The listing builds one solid part. Answer for the finished solid, in the listing's coordinates (mm). A direction names the side the tool comes from. Give positions to 0.01 mm unless a question says otherwise; leave off trailing zeros. Order: outer loops, then holes, each group sorted by start corner. A loop starts at its lowest first (then second) coordinate and runs counter-clockwise, first axis right, second up. Notation, with made-up numbers: (25, 39) -> (38, 39) arc R18 cw to (38, 57) -> close; hole circle Ø5 at (71.5, -17.75). An arc over 180 degrees is marked (long way). Write item = value, one per line. Start each with the question number.
```python
from build123d import *

# Parameters (mm, degrees)
SKETCH1_W                            = 50.8
SKETCH1_H                            = 50.8
BOSS_EXTRUDE1_DEPTH                  = 73.025
CUT_EXTRUDE1_DEPTH                   = 3.175
SKETCH3_R                            = 55.5625
CUT_EXTRUDE2_DEPTH                   = 103.439887861
F_8_32_TAPPED_HOLE1_D                = 3.4544
F_8_32_TAPPED_HOLE1_DEPTH            = 10.70864
F_8_32_TAPPED_HOLE1_TIP              = 1.037806461
F_8_32_TAPPED_HOLE2_D                = 3.4544
F_8_32_TAPPED_HOLE2_DEPTH            = 10.70864
F_8_32_TAPPED_HOLE2_TIP              = 1.037806461
F_10_0_1935_DIAMETER_HOLE1_OUTLINE_R = 2.45745
F_10_0_1935_DIAMETER_HOLE1_DEPTH     = 69.85


# Read off the part's stored shape, not the designer's step: #10 (0.1935) Diameter Hole1
with BuildPart() as part:
    # Sketch1 → Boss-Extrude1 (new body)
    with BuildSketch(Plane(origin=(0, 0, 0), x_dir=(1, 0, 0), z_dir=(0, 1, 0))):
        with Locations((25.4, 25.4)):
            Rectangle(SKETCH1_W, SKETCH1_H)
    extrude(amount=BOSS_EXTRUDE1_DEPTH)

    # Sketch2 → Cut-Extrude1 (cut)
    with BuildSketch(Plane(origin=(0, 73.025, 0), x_dir=(1, 0, 0), z_dir=(0, 1, 0))):
        with BuildLine():
            Line((130.016993909, 125.017737196), (134.25782275, 78.573759143))
            ThreePointArc((134.25782275, 78.573759143), (134.034685181, 75.298190088), (132.798116214, 72.256802214))
            ThreePointArc((132.798116214, 72.256802214), (130.01096738, 66.280890285), (128.580118229, 59.844090402))
            ThreePointArc((128.580118229, 59.844090402), (125.846501332, 47.24207899), (120.576283082, 35.473130329))
            ThreePointArc((120.576283082, 35.473130329), (120.013426501, 34.114565768), (119.824473194, 32.656209898))
            ThreePointArc((119.824473194, 32.656209898), (117.90735564, 28.45485307), (113.469501546, 27.177281171))
            ThreePointArc((113.469501546, 27.177281171), (106.116591491, 23.83727612), (106.198458812, 15.761744078))
            ThreePointArc((106.198458812, 15.761744078), (105.465515747, 8.75311664), (98.443142857, 8.166309094))
            ThreePointArc((98.443142857, 8.166309094), (95.25, 9.168506799), (92.056857143, 8.166309094))
            ThreePointArc((92.056857143, 8.166309094), (88.9, 7.1755), (85.743142857, 8.166309094))
            ThreePointArc((85.743142857, 8.166309094), (82.55, 9.168506799), (79.356857143, 8.166309094))
            ThreePointArc((79.356857143, 8.166309094), (76.212257074, 7.175513597), (73.063291467, 8.152345678))
            ThreePointArc((73.063291467, 8.152345678), (69.907489389, 9.140393728), (66.74574768, 8.171520637))
            ThreePointArc((66.74574768, 8.171520637), (63.508942298, 7.175501389), (60.273525168, 8.176020964))
            ThreePointArc((60.273525168, 8.176020964), (57.10532095, 9.149271709), (53.943097961, 8.156759366))
            ThreePointArc((53.943097961, 8.156759366), (50.791625748, 7.175506347), (47.643142857, 8.166309094))
            ThreePointArc((47.643142857, 8.166309094), (44.45, 9.168506799), (41.256857143, 8.166309094))
            ThreePointArc((41.256857143, 8.166309094), (38.1, 7.1755), (34.943142857, 8.166309094))
            ThreePointArc((34.943142857, 8.166309094), (31.75, 9.168506799), (28.556857143, 8.166309094))
            ThreePointArc((28.556857143, 8.166309094), (25.4, 7.1755), (22.243142857, 8.166309094))
            ThreePointArc((22.243142857, 8.166309094), (19.05, 9.168506799), (15.856857143, 8.166309094))
            ThreePointArc((15.856857143, 8.166309094), (8.793588587, 8.793588587), (8.166309094, 15.856857143))
            ThreePointArc((8.166309094, 15.856857143), (9.168506799, 19.05), (8.166309094, 22.243142857))
            ThreePointArc((8.166309094, 22.243142857), (7.1755, 25.4), (8.166309094, 28.556857143))
            ThreePointArc((8.166309094, 28.556857143), (9.168506799, 31.75), (8.166309094, 34.943142857))
            ThreePointArc((8.166309094, 34.943142857), (7.1755, 38.1), (8.166309094, 41.256857143))
            ThreePointArc((8.166309094, 41.256857143), (9.168506799, 44.45), (8.166309094, 47.643142857))
            ThreePointArc((8.166309094, 47.643142857), (7.175506347, 50.791625748), (8.156759366, 53.943097961))
            ThreePointArc((8.156759366, 53.943097961), (9.149271709, 57.10532095), (8.176020964, 60.273525168))
            ThreePointArc((8.176020964, 60.273525168), (7.175501389, 63.508942298), (8.171520637, 66.74574768))
            ThreePointArc((8.171520637, 66.74574768), (9.140393728, 69.907489389), (8.152345678, 73.063291467))
            ThreePointArc((8.152345678, 73.063291467), (7.175513597, 76.212257074), (8.166309094, 79.356857143))
            ThreePointArc((8.166309094, 79.356857143), (9.168506799, 82.55), (8.166309094, 85.743142857))
            ThreePointArc((8.166309094, 85.743142857), (7.1755, 88.9), (8.166309094, 92.056857143))
            ThreePointArc((8.166309094, 92.056857143), (9.168506799, 95.25), (8.166309094, 98.443142857))
            ThreePointArc((8.166309094, 98.443142857), (8.75311664, 105.465515747), (15.761744078, 106.198458812))
            ThreePointArc((15.761744078, 106.198458812), (23.83727612, 106.116591491), (27.177281171, 113.469501546))
            ThreePointArc((27.177281171, 113.469501546), (28.45485307, 117.90735564), (32.656209898, 119.824473194))
            ThreePointArc((32.656209898, 119.824473194), (34.114565768, 120.013426501), (35.473130329, 120.576283082))
            ThreePointArc((35.473130329, 120.576283082), (47.24207899, 125.846501332), (59.844090402, 128.580118229))
            ThreePointArc((59.844090402, 128.580118229), (68.705211612, 130.952457845), (76.452938417, 135.863689229))
            ThreePointArc((76.452938417, 135.863689229), (80.625736152, 138.0725352), (85.345346996, 138.201045691))
            Line((85.345346996, 138.201045691), (125.626948268, 129.926898817))
            ThreePointArc((125.626948268, 129.926898817), (128.63345164, 128.197989094), (130.016993909, 125.017737196))
        make_face()
    extrude(amount=-CUT_EXTRUDE1_DEPTH, mode=Mode.SUBTRACT)

    # Sketch3 → Cut-Extrude2 (cut, through all)
    with BuildSketch(Plane(origin=(0, 73.025, 0), x_dir=(1, 0, 0), z_dir=(0, 1, 0))):
        with Locations((66.675, 66.675)):
            Circle(SKETCH3_R)
    extrude(amount=-CUT_EXTRUDE2_DEPTH, mode=Mode.SUBTRACT)

    # #8-32 Tapped Hole1
    with Locations(Plane(origin=(393.7, -15.875, 0), x_dir=(1, 0, 0), z_dir=(0, 0, 1))):
        with Locations((-376.782, 41.275)):
            Hole(F_8_32_TAPPED_HOLE1_D / 2, depth=F_8_32_TAPPED_HOLE1_DEPTH)
            with Locations((0, 0, -(F_8_32_TAPPED_HOLE1_DEPTH + F_8_32_TAPPED_HOLE1_TIP / 2))):  # 118° drill point
                Cone(0, F_8_32_TAPPED_HOLE1_D / 2, F_8_32_TAPPED_HOLE1_TIP, mode=Mode.SUBTRACT)

    # #8-32 Tapped Hole2
    with Locations(Plane(origin=(0, -15.875, -393.7), x_dir=(0, 0, 1), z_dir=(-1, 0, 0))):
        with Locations((374.968, 41.275)):
            Hole(F_8_32_TAPPED_HOLE2_D / 2, depth=F_8_32_TAPPED_HOLE2_DEPTH)
            with Locations((0, 0, -(F_8_32_TAPPED_HOLE2_DEPTH + F_8_32_TAPPED_HOLE2_TIP / 2))):  # 118° drill point
                Cone(0, F_8_32_TAPPED_HOLE2_D / 2, F_8_32_TAPPED_HOLE2_TIP, mode=Mode.SUBTRACT)

    # #10 (0.1935) Diameter Hole1 outline → #10 (0.1935) Diameter Hole1 (cut)
    with BuildSketch(Plane(origin=(0, 0, 0), x_dir=(1, 0, 0), z_dir=(0, 1, 0))):
        with Locations((12.7, 12.7)):
            Circle(F_10_0_1935_DIAMETER_HOLE1_OUTLINE_R)
    extrude(amount=F_10_0_1935_DIAMETER_HOLE1_DEPTH, mode=Mode.SUBTRACT)


solid = part.part
```
Item 1: A cutting plane is placed at A-A, the plane y = 52.5. Write down the section's boundary in (x, z) (1 decimal), plus the area to 3 significant figures.
Item 2: Flat-ended cylindrical pins translate along their axes: pin 1 (6.5 mm diameter, centred on x = 12.7, z = -12.7, fed in from +Y); pin 2 (4 mm diameter, centred on y = 28.5, z = -24, fed in from +X); pin 3 (2 mm diameter, centred on x = 16.918, y = 25.4, fed in from -Z). Find the tip coordinate at first contact, or state that the pin passes through.
Item 3: A cutting plane is placed at C-C, the plane x = 24. Write down the section's boundary in (y, z) (3 decimals).
Item 4: Which of the six approach directions +Z, -Z, +X, -X, +Y, -Y give full straight-line access (tool end or side, diameter ignored) to faces 1 (the cylindrical face through (9.17, 71.46, -44.4)), 2 (the cylindrical face through (31.8, 71.46, -9.17)), 3 (the cylindrical face through (27.115, 35.414, -27.66))?
Item 5: The mould has two halves that part along X. Classify faces 4 (the flat face through (19, 0, -20)), 5 (the cylindrical face through (19.1, 71.46, -9.17)), 6 (the flat face through (50.8, 36, -7)): +X half, -X half, draft (parallel to the pull), parting line (faces both ways), or undercut.
Item 6: Consider L1, parallel to Z at x = 8.5, y = 25.4; L2, parallel to X at y = 25.4, z = -6.25; L3, parallel to Y at x = 19.5, z = -33. Determine where each line is inside the solid, lowest interval first. Write a range as from..to.
Item 7: A cutting plane is placed at B-B, the plane z = -43. Write down the section's boundary in (x, y) (3 decimals), plus the area to 3 significant figures.
Check values:
q1.outline = (0, -50.8) -> (13.4, -50.8) arc R55.6 cw to (50.8, -13.4) -> (50.8, 0) -> (0, 0) -> close; hole circle Ø4.9 at (12.7, -12.7)
q1.area = 1,620 mm^2
q2.pin_1 = 69.85
q2.pin_2 = 33.64
q2.pin_3 = -44.07
q3.outline = (0, -31.094) -> (69.85, -31.094) -> (69.85, -7.356) -> (73.025, -7.356) -> (73.025, 0) -> (0, 0) -> close
q4.face_1 = +X, +Y
q4.face_2 = -Z, +Y
q4.face_3 = -Z, +X, +Y, -Y
q5.face_4 = draft
q5.face_5 = undercut
q5.face_6 = +X half
q6.L1 = -50.8..-20.46, -17..0
q6.L2 = 0..15.19, 18.65..50.8
q6.L3 = 0..69.85
q7.outline = (0, 0) -> (16.409, 0) -> (16.409, 69.85) -> (8.977, 69.85) -> (8.977, 73.025) -> (0, 73.025) -> close
q7.area = 1,170 mm^2
